Can you work these out from the drawing? Everything is in mm from the part's minimum corner. Round coordinates to 2 decimals unless told otherwise and drop trailing zeros. Order: outer loops, then holes, each group sorted by start corner. A loop starts at its lowest first (then second) coordinate and runs counter-clockwise, first axis right, second up. Notation, with made-up numbers: M 72,49.25 L 85,49.25 A20 cw 85,69.25 Z; hole C 19,51 d4. An arc over 180 degrees is marked long. Answer as CSV lines item,"result". Start each with the question number.
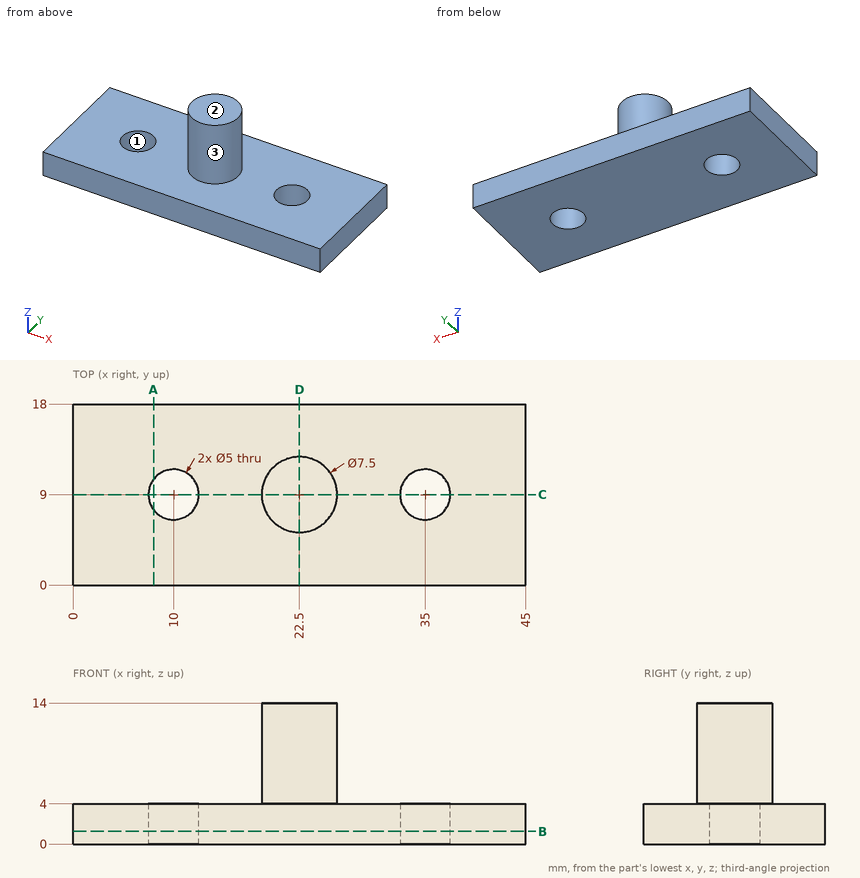
(1) I'm going to push flat-ended pins straight in: P1, Ø5.5, axis at x = 28.5, y = 12, coming from the +Z side; P2, Ø3, axis at y = 8, z = 8.5, coming from the -X side. Where does each tip first touch, or does it pass through?
(2) I want a section at A-A on x = 8. Write out the boundary of the cut face in (y, z), and give its area (3 significant figures).
(3) If we mould it in two halves opening along Y, with no side actions, what happens to the marked faces 1, 2 and 3? For each: +Y half, -Y half, draft (parallel to the pull), parting line (faces both ways), or undercut.
(4) I want a section at D-D on x = 22.5. Write out the boundary of the cut face in (y, z).
(5) If I drill on line 1 along Y through (x, z) = (10, 3.15); line 2 along Z through (x, y) = (4.5, 8.25); line 3 along X through (y, z) = (9.5, 10.25), over which ranges is the centre line in solid material (lowest first)?
(6) I want a section at C-C on y = 9. Write out the boundary of the cut face in (x, z), and give its area (3 significant figures).
(7) I want a section at B-B on z = 1.25. Write out the boundary of the cut face in (x, y), and give its area (3 significant figures).
From the geometry:
1,P1,"z = 4"
1,P2,"x = 18.75"
2,outline,"M 0,0 L 7.5,0 L 7.5,4 L 0,4 Z; M 10.5,0 L 18,0 L 18,4 L 10.5,4 Z"
2,area,"60.0 mm²"
3,face 1,"undercut"
3,face 2,"draft"
3,face 3,"parting line"
4,outline,"M 0,0 L 18,0 L 18,4 L 12.75,4 L 12.75,14 L 5.25,14 L 5.25,4 L 0,4 Z"
5,line 1,"0 to 6.5, 11.5 to 18"
5,line 2,"0 to 4"
5,line 3,"18.78 to 26.22"
6,outline,"M 0,0 L 7.5,0 L 7.5,4 L 0,4 Z; M 12.5,0 L 32.5,0 L 32.5,4 L 26.25,4 L 26.25,14 L 18.75,14 L 18.75,4 L 12.5,4 Z; M 37.5,0 L 45,0 L 45,4 L 37.5,4 Z"
6,area,"215 mm²"
7,outline,"M 0,0 L 45,0 L 45,18 L 0,18 Z; hole C 10,9 d5; hole C 35,9 d5"
7,area,"771 mm²"
